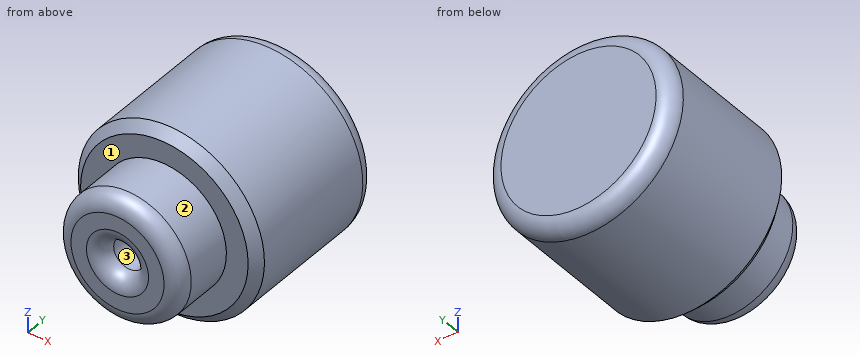
```python
from build123d import *

# Parameters (mm, degrees)
F0_W    = 20
F0_H    = 15
F0_W_2  = 42.9629645813
F2_SIZE = 3
F3_R    = 5


with BuildPart() as f1:
    # F0 (on Right) → F1 (revolve)
    with BuildSketch(Plane.YZ):
        with Locations((-60, 12.5)):
            Rectangle(F0_W, F0_H)
        Polygon((0, 30), (-50, 30), (-50, 20), (-7.0370354187, 20), (-7.0370354187, 5), (-50, 5), (-50, 0), (0, 0), align=None)
        with Locations((-28.5185177093, 12.5)):
            Rectangle(F0_W_2, F0_H)
    revolve(axis=Axis((0, -25, 0), (0, 1, 0)))

    # F2
    f2_edges = [f1.edges().sort_by_distance(p)[0] for p in [
        (0, -50, -30),
    ]]
    chamfer(f2_edges, length=F2_SIZE)

    # F3
    f3_edges = [f1.edges().sort_by_distance(p)[0] for p in [
        (0, -70, -20),
        (0, -70, -5),
        (0, 0, -30),
    ]]
    fillet(f3_edges, radius=F3_R)


solid = f1.part
```
Can you work these out from the model? Positions are in its coordinate system, mm. Face numbers are marked on the shaded views. Give positions to 0.01 mm unless a question says otherwise; leave off trailing zeros. Loops run counter-clockwise (first coordinate to the right, second up) from the corner with the lowest first, then second, coordinate; pieces in that order, holes last. Notation, with made-up numbers: M -33.75,26.5 L 3.25,26.5 A16 ccw 3.25,45.5 Z; hole C 6,43 d1. An arc over 180 degrees is marked long. Use one line per item in the form item = value. Start each with the question number.
(1) I want a section at A-A, the plane z = 0. Write out the boundary of the cut face in (x, y).
(2) I'm going to push flat-ended pins straight in: P1, Ø12, axis at x = -19.5, y = -57, coming from the +Z side; P2, Ø3, axis at y = -44.5, z = -0.5, coming from the +X side; P3, Ø5, axis at x = -19, z = -5, coming from the -Y side. Where does each tip first touch, or does it pass through?
(3) Please list where these lines run through material, in increasing order: line 1 (X direction, y = -58.75, z = 0); line 2 (Y direction, x = 15, z = 16.5); line 3 (X direction, y = -67, z = -5).
(4) Thinking about a two-plate mould opening in X: for the marked faces 1, 2 and 3, which applies, released by +X, released by -X, zero draft, split by the parting line, or undercut?
(5) I want a section at B-B, the plane y = -63. Write out the boundary of the cut face in (x, z).
(6) I want a section at D-D, the plane y = -41. Write out the boundary of the cut face in (x, z), and give its area (3 significant figures).
(7) I want a section at C-C, the plane x = 0. Write out the boundary of the cut face in (y, z), and give its area (3 significant figures).
Worked out:
q1.outline = M -30,-47 L -27,-50 L -20,-50 L -20,-65 A5 ccw -15,-70 L -10,-70 A5 ccw -5,-65 L -5,-50 L 5,-50 L 5,-65 A5 ccw 10,-70 L 15,-70 A5 ccw 20,-65 L 20,-50 L 27,-50 L 30,-47 L 30,-5 A5 ccw 25,0 L -25,0 A5 ccw -30,-5 Z
q2.P1 = 14.76
q2.P2 = 30
q2.P3 = -69.52
q3.line_1 = -20 to -5, 5 to 20
q3.line_2 = -50 to 0
q3.line_3 = -18.93 to -2.09, 2.09 to 18.93
q4.face_1 = zero draft
q4.face_2 = split by the parting line
q4.face_3 = undercut
q5.outline = C 0,0 d40; hole C 0,0 d10
q6.outline = C 0,0 d60
q6.area = 2,830 mm²
q7.outline = M -70,-15 A5 ccw -65,-20 L -50,-20 L -50,-27 L -47,-30 L -5,-30 A5 ccw 0,-25 L 0,25 A5 ccw -5,30 L -47,30 L -50,27 L -50,20 L -65,20 A5 ccw -70,15 L -70,10 A5 ccw -65,5 L -50,5 L -50,-5 L -65,-5 A5 ccw -70,-10 Z
q7.area = 3,560 mm²
